For this review, use the dimensioned drawing (mm, ordinates from the lowest corner) and the shaded views. Give positions to 0.01 mm unless a question says otherwise; leave off trailing zeros. Write each loop counter-clockwise with the first axis right and the second up, starting at its lowest first coordinate (ties: lowest second). Pieces come first, ordered by that corner, then holes. Notation, with made-up numbers: M 56,38 L 65,38 A23 ccw 65,73 Z; hole C -21,6 d11. An arc over 180 degrees is marked long. One line per item, written item: value. Start each with the question number.
Item 1: Consider section A-A, the plane x = 18. Write out the cut boundary in (y, z), and give its area (3 significant figures).
Item 2: Consider section D-D, the plane x = 7. Write out the cut boundary in (y, z).
Item 3: Mouldability with a two-part tool opening along Y and no side actions: class the marked faces 1 and 2 as released by +Y, released by -Y, zero draft, split by the parting line, or undercut.
Item 4: Clearance check with flat-ended pins moving along their axes: pin 1 Ø5 at (y, z) = (14, 15.5) entering from -X; pin 2 Ø12.5 at (x, z) = (24.5, 36.5) entering from -Y; pin 3 Ø5.5 at (x, y) = (20, 53.5) entering from +Z. State where each tip first meets the part, or that it passes through.
Item 5: To check wall thickness, follow probe 1 along X at (y, z) = (29, 9); probe 2 along Y at (x, z) = (27, 46.5); probe 3 along Y at (x, z) = (6, 7.5). State the ranges of each line that lie inside material, in increasing order.
Item 6: Consider section C-C, the plane z = 35. Write out the cut boundary in (x, y).
Item 7: Consider section B-B, the plane y = 43.5. Write out the cut boundary in (x, z), and give its area (3 significant figures).
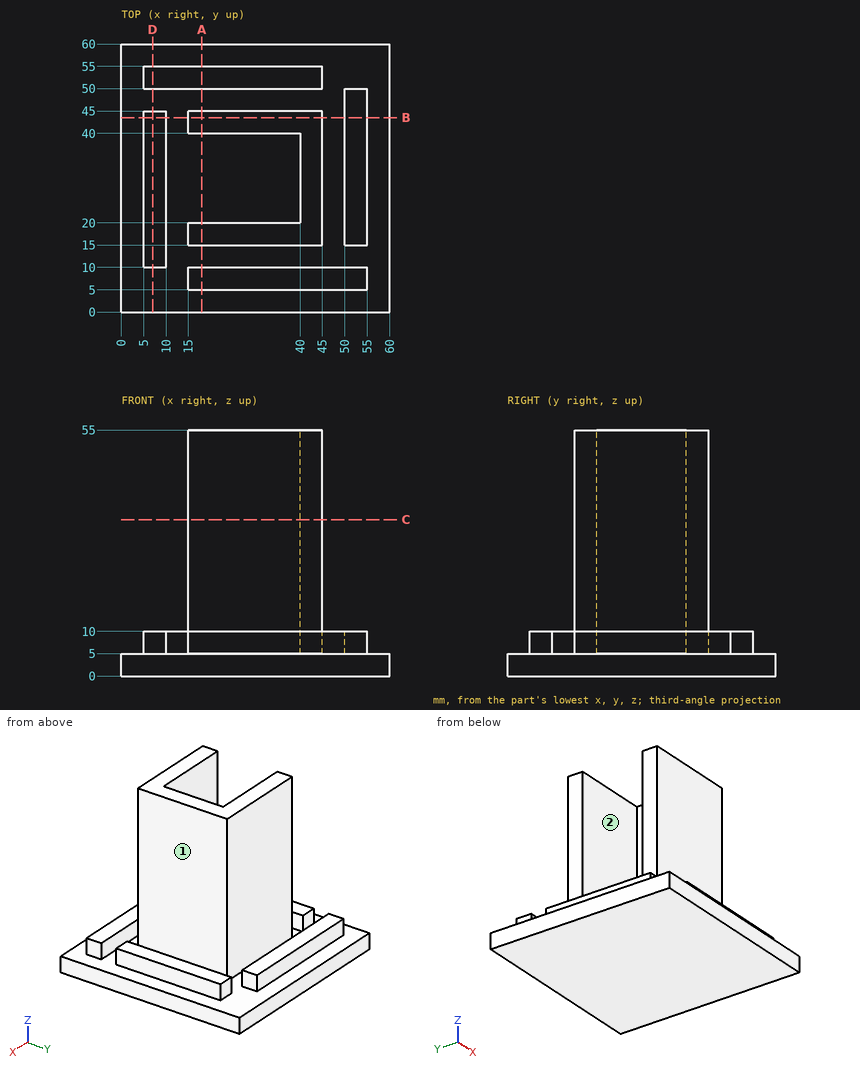
Model answer:
1. outline: M 0,0 L 60,0 L 60,5 L 55,5 L 55,10 L 50,10 L 50,5 L 45,5 L 45,55 L 40,55 L 40,5 L 20,5 L 20,55 L 15,55 L 15,5 L 10,5 L 10,10 L 5,10 L 5,5 L 0,5 Z
1. area: 850 mm2
2. outline: M 0,0 L 60,0 L 60,5 L 55,5 L 55,10 L 50,10 L 50,5 L 45,5 L 45,10 L 10,10 L 10,5 L 0,5 Z
3. face 1: zero draft
3. face 2: undercut
4. pin 1: stops at x = 15
4. pin 2: stops at y = 15
4. pin 3: stops at z = 10
5. probe 1: x = 5 to 10, 40 to 45, 50 to 55
5. probe 2: y = 15 to 20, 40 to 45
5. probe 3: y = 10 to 45, 50 to 55
6. outline: M 15,15 L 45,15 L 45,45 L 15,45 L 15,40 L 40,40 L 40,20 L 15,20 Z
7. outline: M 0,0 L 60,0 L 60,5 L 55,5 L 55,10 L 50,10 L 50,5 L 45,5 L 45,55 L 15,55 L 15,5 L 10,5 L 10,10 L 5,10 L 5,5 L 0,5 Z
7. area: 1,850 mm2
